from build123d import *

# Parameters (mm, degrees)
L_ANGLE_EQUAL_40X40X3_2_DEPTH = 1920
SKETCH15_R                    = 2
CUT_EXTRUDE1_DEPTH            = 10
SKETCH16_R                    = 2
CUT_EXTRUDE2_DEPTH            = 3


with BuildPart() as part:
    # Sketch13 → L angle (equal) 40X40X3(2) (new body)
    with BuildSketch(Plane(origin=(0, 0, 0), x_dir=(0, 0, -1), z_dir=(1, 0, 0))):
        with BuildLine():
            Line((0, 40), (0, 0))
            Line((0, 0), (40, 0))
            ThreePointArc((40, 0), (39.121320344, 2.121320344), (37, 3))
            Line((37, 3), (9, 3))
            ThreePointArc((9, 3), (4.757359313, 4.757359313), (3, 9))
            Line((3, 9), (3, 37))
            ThreePointArc((3, 37), (2.121320344, 39.121320344), (0, 40))
        make_face()
    extrude(amount=L_ANGLE_EQUAL_40X40X3_2_DEPTH)

    # Sketch15 → Cut-Extrude1 (cut)
    with BuildSketch(Plane(origin=(0, 0, 0), x_dir=(-1, 0, 0), z_dir=(0, -1, 0))):
        with Locations(Location((-960, 20, 0), (0, 0, 90))):
            Circle(SKETCH15_R)
        with Locations(Location((-470, 20, 0), (0, 0, 90))):
            Circle(SKETCH15_R)
        with Locations(Location((-1450, 20, 0), (0, 0, 90))):
            Circle(SKETCH15_R)
    extrude(amount=-CUT_EXTRUDE1_DEPTH, mode=Mode.SUBTRACT)

    # Sketch16 → Cut-Extrude2 (cut)
    with BuildSketch(Plane.XY):
        with Locations((960, 20)):
            Circle(SKETCH16_R)
        with Locations((1450, 20)):
            Circle(SKETCH16_R)
        with Locations((470, 20)):
            Circle(SKETCH16_R)
    extrude(amount=-CUT_EXTRUDE2_DEPTH, mode=Mode.SUBTRACT)


solid = part.part
Input: part model. Units: mm. Frame: model coordinates. Give positions to 0.01 mm unless a question says otherwise; leave off trailing zeros. Write each loop counter-clockwise with the first axis right and the second up, starting at its lowest first coordinate (ties: lowest second). Pieces come first, ordered by that corner, then holes. Notation, with made-up numbers: (57.5, 85.25) -> (107.5, 85.25) arc R31 ccw to (107.5, 112.25) -> close; hole circle Ø5 at (24.5, -17.5). An arc over 180 degrees is marked (long way). Use one line per item in the form item = value. Start each with the question number.
1) Section query B-B on z = -28. Return the cut outline in (x, y), then the cut area to 3 significant figures.
2) Section query A-A on x = 1375. Return the cut outline in (y, z).
3) Pin query (flat end, axial travel): pin 1 (2.5 mm diameter, centred on x = 960, y = 20, fed in from -Z); pin 2 (22.5 mm diameter, centred on x = 1101.5, y = 27.5, fed in from -Z); pin 3 (6 mm diameter, centred on x = 903.5, z = -31, fed in from +Y); pin 4 (10 mm diameter, centred on x = 323.5, y = 6.5, fed in from -Z). Return the tip coordinate at first contact, or that it passes through.
4) Ray query, probe 1 along Z at (x, y) = (470, 0.85); probe 2 along Y at (x, z) = (282.5, -32); probe 3 along Z at (x, y) = (264.5, 13). Return the intervals inside material, ascending. Write a range as from..to.
Outcome:
q1.outline = (0, 0) -> (1920, 0) -> (1920, 3) -> (0, 3) -> close
q1.area = 5,760 mm^2
q2.outline = (0, -40) arc R3 ccw to (3, -37) -> (3, -9) arc R6 cw to (9, -3) -> (37, -3) arc R3 ccw to (40, 0) -> (0, 0) -> close
q3.pin_1 = through
q3.pin_2 = -3
q3.pin_3 = 3
q3.pin_4 = -39.6
q4.probe_1 = -39.88..-22, -18..0
q4.probe_2 = 0..3
q4.probe_3 = -3..0
